```python
from build123d import *

# Parameters (mm, degrees)
CUT_EXTRUDE1_START = 2.2987
CUT_EXTRUDE1_DEPTH = 10.922
CIRPATTERN1_COUNT  = 10
SKETCH4_R          = 2.0828
CUT_EXTRUDE2_DEPTH = 19.796832346
CUT_EXTRUDE3_DEPTH = 1.5621
CIRPATTERN2_COUNT  = 2
CIRPATTERN2_ANGLE  = 90


with BuildPart() as part:
    # Sketch2 → Revolve1 (revolve)
    with BuildSketch(Plane(origin=(0, 0, 0), x_dir=(0, 0, -1), z_dir=(1, 0, 0)), mode=Mode.PRIVATE) as revolve1_sk:
        with BuildLine():
            Line((-10.3124, 3.175), (10.3124, 3.175))
            Line((10.3124, 3.175), (10.3124, 11.1125))
            Line((10.3124, 11.1125), (9.46785, 11.1125))
            ThreePointArc((9.46785, 11.1125), (8.846862309, 10.395787163), (8.6233, 9.4742))
            Line((8.6233, 9.4742), (8.6233, 7.8359))
            Line((8.6233, 7.8359), (-2.2987, 7.8359))
            Line((-2.2987, 7.8359), (-2.2987, 9.4742))
            ThreePointArc((-2.2987, 9.4742), (-2.522262309, 10.395787163), (-3.14325, 11.1125))
            Line((-3.14325, 11.1125), (-3.9878, 11.1125))
            Line((-3.9878, 11.1125), (-3.9878, 5.5499))
            Line((-3.9878, 5.5499), (-10.3124, 5.5499))
            Line((-10.3124, 5.5499), (-10.3124, 3.175))
        make_face()
    revolve(revolve1_sk.sketch.rotate(Axis((0, 0, 10.3124), (0, 0, -1)), 90), axis=Axis((0, 0, 10.3124), (0, 0, -1)))

    # Sketch3 → Cut-Extrude1 (cut)
    with BuildSketch(Plane.XY.offset(CUT_EXTRUDE1_START)):
        with BuildLine():
            Line((-0.635, 6.329348022), (0.635, 6.329348022))
            Line((0.635, 6.329348022), (1.287830721, 7.729348022))
            ThreePointArc((1.287830721, 7.729348022), (0, 7.8359), (-1.287830721, 7.729348022))
            Line((-1.287830721, 7.729348022), (-0.635, 6.329348022))
        make_face()
    cut_extrude1 = extrude(amount=-CUT_EXTRUDE1_DEPTH, mode=Mode.SUBTRACT)

    # CirPattern1: Cut-Extrude1 ×10 about axis
    cirpattern1_axis = Axis((0, 0, 0), (0, 0, 1))
    for i in range(1, CIRPATTERN1_COUNT):
        add(cut_extrude1.rotate(cirpattern1_axis, i * 360 / CIRPATTERN1_COUNT), mode=Mode.SUBTRACT)

    # Sketch4 → Cut-Extrude2 (cut, through all)
    with BuildSketch(Plane(origin=(0, 0, 0), x_dir=(1, 0, 0), z_dir=(0, 1, 0))):
        with Locations(Location((0, -7.1501, 0), (0, 0, 90))):
            Circle(SKETCH4_R)
    cut_extrude2 = extrude(amount=CUT_EXTRUDE2_DEPTH, mode=Mode.SUBTRACT)

    # Sketch5 → Revolve2 (revolve)
    with BuildSketch(Plane.XY.offset(7.1501), mode=Mode.PRIVATE) as revolve2_sk:
        Polygon((1.5748, 5.144252538), (2.0828, 4.636252538), (2.0828, 3.81), (1.4478, 3.175), (0, 3.175), (0, 5.144252538), align=None)
    revolve2 = revolve(revolve2_sk.sketch.rotate(Axis((0, 0, 7.1501), (0, 1, 0)), 90), axis=Axis((0, 0, 7.1501), (0, 1, 0)))

    # Sketch6 → Cut-Extrude3 (cut)
    with BuildSketch(Plane(origin=(0, 5.144252538, 0), x_dir=(1, 0, 0), z_dir=(0, 1, 0))):
        Polygon((0, -5.947594859), (-1.0414, -6.54884743), (-1.0414, -7.75135257), (0, -8.352605141), (1.0414, -7.75135257), (1.0414, -6.54884743), align=None)
    cut_extrude3 = extrude(amount=-CUT_EXTRUDE3_DEPTH, mode=Mode.SUBTRACT)

    # CirPattern2: Cut-Extrude2, Revolve2, Cut-Extrude3 ×2 about axis
    cirpattern2_axis = Axis((0, 0, 0), (0, 0, -1))
    add([cut_extrude2.rotate(cirpattern2_axis, i * CIRPATTERN2_ANGLE / (CIRPATTERN2_COUNT - 1)) for i in range(1, CIRPATTERN2_COUNT)], mode=Mode.SUBTRACT)
    add([revolve2.rotate(cirpattern2_axis, i * CIRPATTERN2_ANGLE / (CIRPATTERN2_COUNT - 1)) for i in range(1, CIRPATTERN2_COUNT)])
    add([cut_extrude3.rotate(cirpattern2_axis, i * CIRPATTERN2_ANGLE / (CIRPATTERN2_COUNT - 1)) for i in range(1, CIRPATTERN2_COUNT)], mode=Mode.SUBTRACT)


solid = part.part
```
Source: CAD feature listing. Evaluate the final solid. Frame: model axes, mm. A direction names the side the tool comes from. Coordinates: 2 decimals unless noted, no trailing zeros. Loops run counter-clockwise (first coordinate to the right, second up) from the corner with the lowest first, then second, coordinate; pieces in that order, holes last. Notation, with made-up numbers: M 88,-9.75 L 124,-9.75 A13 ccw 124,-5.75 Z; hole C 57.25,86 d10. An arc over 180 degrees is marked long. Put each result on its own line as item: value. Start each with the question number.
1) Contact query for flat-ended pins moving along their axis: pin 1 Ø4 at (x, z) = (7, 7.5) entering from -Y; pin 2 Ø2.5 at (y, z) = (0, 7) entering from -X; pin 3 Ø10 at (y, z) = (-8, -4.5) entering from -X. Output: stop coordinate, or through.
2) Cut plane A-A on z = 4.5. Return the cut outline in (x, y) (3 decimals).
3) Ray query, L1, parallel to Y at x = 0, z = -2.75 (3 decimals); L2, parallel to Z at x = -0.5, y = -7.75; L3, parallel to Y at x = 6.5, z = -5.75. Return the intervals inside material, ascending. Write a range as from..to.
4) Reachability of faces 3 (the face through (4.37, 0.51, 6.24)), 4 (the face through (2.406, 7.457, -3.086)), 5 (the face through (-1.041, 4, 7)), 6 (the face through (3.71, 5.13, -3.09)), 7 (the face through (-4.9, -5.117, -3.086)) from +Z, -Z, +X, -X, +Y, -Y: full face, straight path, thin tool, end or side. Return the list, or none.
5) Pull-direction query (Z, two-part tool) for faces 1 (the face through (3.727, -5.115, -3.086)), 2 (the face through (-8.2, -7.5, 3.6)); classes: pulls with the +Z half, pulls with the -Z half, needs draft (parallel to the pull), parting line crosses it, or undercut.
The answers:
1. pin 1: stops at y = -2.41
1. pin 2: stops at x = -5.55
1. pin 3: stops at x = -8.92
2. outline: C 0,0 d11.1; hole C 0,0 d6.35
3. L1: y = -6.329..-3.175, 3.175..6.329
3. L2: z = -10.31..-8.62, 2.3..3.99
3. L3: y = -4.38..-3.19, -1.32..1.32, 3.19..4.38
4. face 3: +X
4. face 4: +X, +Y
4. face 5: +Y
4. face 6: none
4. face 7: -Y
5. face 1: undercut
5. face 2: needs draft
